Verification items for the finished model (mm, model axes). Round coordinates to 2 decimals unless told otherwise and drop trailing zeros. Loops run counter-clockwise (first coordinate to the right, second up) from the corner with the lowest first, then second, coordinate; pieces in that order, holes last. Notation, with made-up numbers: (-10, -8) -> (17, -8) arc R17 cw to (17, 17) -> close; hole circle Ø8 at (-30, 15). An arc over 180 degrees is marked (long way). Use a Markdown table: item, result. Add a question column.
```python
from build123d import *

# Parameters (mm, degrees)
CROQUIS1_R              = 2
CROQUIS1_R_2            = 84.42
CROQUIS1_R_3            = 80.42
SALIENTE_EXTRUIR1_DEPTH = 3


with BuildPart() as part:
    # Croquis1 → Saliente-Extruir1 (new body)
    # profile 1 of 3: a face of its own
    with BuildSketch(Plane(origin=(0, 0, 0), x_dir=(1, 0, 0), z_dir=(0, 1, 0))):
        with BuildLine():
            Line((83.93888491, -9), (97, -9))
            Line((97, -9), (97, 9))
            Line((97, 9), (83.93888491, 9))
            ThreePointArc((83.93888491, 9), (84.299635421, 4.506425183), (84.42, 0))
            ThreePointArc((84.42, 0), (84.299635421, -4.506425183), (83.93888491, -9))
        make_face()
        with Locations(Location((90, -5, 0), (0, 0, 270))):
            Circle(CROQUIS1_R, mode=Mode.SUBTRACT)
        with Locations(Location((90, 5, 0), (0, 0, 270))):
            Circle(CROQUIS1_R, mode=Mode.SUBTRACT)
    # profile 2 of 3: a face of its own
    with BuildSketch(Plane(origin=(0, 0, 0), x_dir=(1, 0, 0), z_dir=(0, 1, 0))):
        Circle(CROQUIS1_R_2)
        with Locations(Location((0, 0, 0), (0, 0, 270))):
            Circle(CROQUIS1_R_3, mode=Mode.SUBTRACT)
    # profile 3 of 3: a face of its own
    with BuildSketch(Plane(origin=(0, 0, 0), x_dir=(1, 0, 0), z_dir=(0, 1, 0))):
        with BuildLine():
            Line((-97, -9), (-83.93888491, -9))
            ThreePointArc((-83.93888491, -9), (-84.42, 0), (-83.93888491, 9))
            Line((-83.93888491, 9), (-97, 9))
            Line((-97, 9), (-97, -9))
        make_face()
        with Locations(Location((-90, -5, 0), (0, 0, 270))):
            Circle(CROQUIS1_R, mode=Mode.SUBTRACT)
        with Locations(Location((-90, 5, 0), (0, 0, 270))):
            Circle(CROQUIS1_R, mode=Mode.SUBTRACT)
    extrude(amount=SALIENTE_EXTRUIR1_DEPTH)


solid = part.part
```
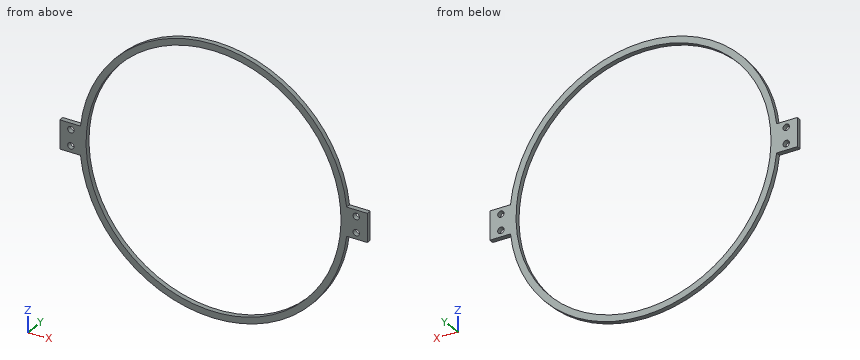
1) Sectioned sample at A-A on x = 0. Enter the section's corners in (y, z).
2) Go/stop test with flat-tipped pins: pin 1 (1.5 mm diameter, centred on x = -91, y = 1.5, fed in from -Z); pin 2 (3.5 mm diameter, centred on x = 90, z = -5, fed in from +Y); pin 3 (1 mm diameter, centred on x = 32.5, y = 2.5, fed in from +Z); pin 4 (1 mm diameter, centred on x = -66.5, y = 1.5, fed in from +Z). Record where each tip stops, or that it passes through.
3) Sectioned sample at B-B on z = 0. Enter the section's corners in (x, y).
4) Thickness scan on line 1 (X direction, y = 1.6, z = -5); line 2 (X direction, y = 0.75, z = 4.5); line 3 (X direction, y = 1.3, z = 37). Record the ranges inside material, lowest first.
5) Sectioned sample at C-C on y = 2.4. Enter the section's corners in (x, z).
Geometry results:
| question | item | result |
|---|---|---|
| 1 | outline | (0, -84.42) -> (3, -84.42) -> (3, -80.42) -> (0, -80.42) -> close; (0, 80.42) -> (3, 80.42) -> (3, 84.42) -> (0, 84.42) -> close |
| 2 | pin 1 | z = -9 |
| 2 | pin 2 | through |
| 2 | pin 3 | z = 78.12 |
| 2 | pin 4 | z = 52.64 |
| 3 | outline | (-97, 0) -> (-80.42, 0) -> (-80.42, 3) -> (-97, 3) -> close; (80.42, 0) -> (97, 0) -> (97, 3) -> (80.42, 3) -> close |
| 4 | line 1 | -97 to -92, -88 to -80.26, 80.26 to 88, 92 to 97 |
| 4 | line 2 | -97 to -91.94, -88.06 to -80.29, 80.29 to 88.06, 91.94 to 97 |
| 4 | line 3 | -75.88 to -71.4, 71.4 to 75.88 |
| 5 | outline | (-97, -9) -> (-83.94, -9) arc R84.42 ccw to (83.94, -9) -> (97, -9) -> (97, 9) -> (83.94, 9) arc R84.42 ccw to (-83.94, 9) -> (-97, 9) -> close; hole circle Ø4 at (-90, -5); hole circle Ø4 at (-90, 5); hole circle Ø160.84 at (0, 0); hole circle Ø4 at (90, -5); hole circle Ø4 at (90, 5) |
